Work out the finished part from the listing and answer in its coordinate system (mm). Coordinates: 2 decimals unless noted, no trailing zeros. Order: outer loops, then holes, each group sorted by start corner. A loop starts at its lowest first (then second) coordinate and runs counter-clockwise, first axis right, second up. Notation, with made-up numbers: M 50.5,-8.5 L 94.5,-8.5 A21 ccw 94.5,5.5 Z; hole C 38.5,87 d6. An arc over 180 degrees is marked long. Use a Markdown table: item, result.
from build123d import *

# Parameters (mm, degrees)
SKETCH1_W                = 110
SKETCH1_H                = 190
BOSS_EXTRUDE1_DEPTH      = 6
CUT_EXTRUDE1_REACH       = 111.936
SKETCH2_R                = 13
CUT_EXTRUDE2_REACH       = 111.936
SKETCH3_R                = 4.1
FILLET1_R                = 3
M4_CLEARANCE_HOLE1_D     = 4.2
M4_CLEARANCE_HOLE1_DEPTH = 19.75
M4_CLEARANCE_HOLE1_TIP   = 1.2618073


with BuildPart() as part:
    # Sketch1 → Boss-Extrude1 (new body)
    with BuildSketch(Plane.XY):
        Rectangle(SKETCH1_W, SKETCH1_H)
    extrude(amount=BOSS_EXTRUDE1_DEPTH)

    # Sketch2 → Cut-Extrude1 (cut, up to next)
    with BuildSketch(Plane.XY.offset(6), mode=Mode.PRIVATE) as cut_extrude1_sk1:
        Circle(SKETCH2_R)
    cut_extrude1_tool1 = extrude(cut_extrude1_sk1.sketch, amount=-CUT_EXTRUDE1_REACH, mode=Mode.PRIVATE) & part.part
    add(cut_extrude1_tool1.solids().sort_by_distance((0, 0, 6))[0], mode=Mode.SUBTRACT)

    # Sketch3 → Cut-Extrude2 (cut, up to next)
    with BuildSketch(Plane.XY.offset(6), mode=Mode.PRIVATE) as cut_extrude2_sk1:
        with Locations((-35, 75)):
            Circle(SKETCH3_R)
    cut_extrude2_tool1 = extrude(cut_extrude2_sk1.sketch, amount=-CUT_EXTRUDE2_REACH, mode=Mode.PRIVATE) & part.part
    # Sketch3 → Cut-Extrude2 (cut, up to next)
    with BuildSketch(Plane.XY.offset(6), mode=Mode.PRIVATE) as cut_extrude2_sk2:
        with Locations((35, 75)):
            Circle(SKETCH3_R)
    cut_extrude2_tool2 = extrude(cut_extrude2_sk2.sketch, amount=-CUT_EXTRUDE2_REACH, mode=Mode.PRIVATE) & part.part
    # Sketch3 → Cut-Extrude2 (cut, up to next)
    with BuildSketch(Plane.XY.offset(6), mode=Mode.PRIVATE) as cut_extrude2_sk3:
        with Locations((35, -75)):
            Circle(SKETCH3_R)
    cut_extrude2_tool3 = extrude(cut_extrude2_sk3.sketch, amount=-CUT_EXTRUDE2_REACH, mode=Mode.PRIVATE) & part.part
    # Sketch3 → Cut-Extrude2 (cut, up to next)
    with BuildSketch(Plane.XY.offset(6), mode=Mode.PRIVATE) as cut_extrude2_sk4:
        with Locations((-35, -75)):
            Circle(SKETCH3_R)
    cut_extrude2_tool4 = extrude(cut_extrude2_sk4.sketch, amount=-CUT_EXTRUDE2_REACH, mode=Mode.PRIVATE) & part.part
    add(cut_extrude2_tool1.solids().sort_by_distance((-35, 75, 6))[0], mode=Mode.SUBTRACT)
    add(cut_extrude2_tool2.solids().sort_by_distance((35, 75, 6))[0], mode=Mode.SUBTRACT)
    add(cut_extrude2_tool3.solids().sort_by_distance((35, -75, 6))[0], mode=Mode.SUBTRACT)
    add(cut_extrude2_tool4.solids().sort_by_distance((-35, -75, 6))[0], mode=Mode.SUBTRACT)

    # Fillet1
    fillet1_edges = [part.edges().sort_by_distance(p)[0] for p in [
        (55, -95, 3),
        (-55, -95, 3),
        (-55, 95, 3),
        (55, 95, 3),
    ]]
    fillet(fillet1_edges, radius=FILLET1_R)

    # M4 Clearance Hole1
    with Locations(Plane(origin=(-12, 12, 6), x_dir=(1, 0, 0), z_dir=(0, 0, 1))):
        with Locations((0, 0), (24, 0), (24, -24), (0, -24)):
            Hole(M4_CLEARANCE_HOLE1_D / 2, depth=M4_CLEARANCE_HOLE1_DEPTH)
            with Locations((0, 0, -(M4_CLEARANCE_HOLE1_DEPTH + M4_CLEARANCE_HOLE1_TIP / 2))):  # 118° drill point
                Cone(0, M4_CLEARANCE_HOLE1_D / 2, M4_CLEARANCE_HOLE1_TIP, mode=Mode.SUBTRACT)


solid = part.part
1. For a pull along X with two mould halves and no side action, classify faces 1 (the face through (-1, 22, 0)), 2 (the face through (-55, -1, 3)), 3 (the face through (-10.316, -7.91, 3.042)) as +X half, -X half, draft (parallel to the pull), parting line (faces both ways), or undercut.
Answers below:
| item | result |
|---|---|
| face 1 | draft |
| face 2 | -X half |
| face 3 | undercut |
2. Section A-A on x = 0 is taken. Determine the outline of the cut face in (y, z).
Answers below:
| item | result |
|---|---|
| outline | M -95,0 L -13,0 L -13,6 L -95,6 Z; M 13,0 L 95,0 L 95,6 L 13,6 Z |
3. Section B-B on y = 75 is taken. Determine the outline of the cut face in (x, z), then the cut area to 3 significant figures.
Answers below:
| item | result |
|---|---|
| outline | M -55,0 L -39.1,0 L -39.1,6 L -55,6 Z; M -30.9,0 L 30.9,0 L 30.9,6 L -30.9,6 Z; M 39.1,0 L 55,0 L 55,6 L 39.1,6 Z |
| area | 562 mm² |
4. Section D-D on y = 0 is taken. Determine the outline of the cut face in (x, z).
Answers below:
| item | result |
|---|---|
| outline | M -55,0 L -13,0 L -13,6 L -55,6 Z; M 13,0 L 55,0 L 55,6 L 13,6 Z |
5. Section C-C on z = 2.45 is taken. Give the number of separate pieces and of enclosed holes in the cut face, then the cut area to 3 significant figures.
Answers below:
| item | result |
|---|---|
| separate pieces | 1 |
| enclosed holes | 9 |
| area | 20,100 mm² |
6. Flat-ended cylindrical pins translate along their axes: P1, Ø7.5, axis at x = 35, y = 75, coming from the -Z side; P2, Ø8, axis at x = -40, y = -13, coming from the -Z side. Find the tip coordinate at first contact, or state that the pin passes through.
Answers below:
| item | result |
|---|---|
| P1 | through |
| P2 | z = 0 |
7. Find the intervals of material crossed by probe 1 along Y at (x, z) = (-35, 1.3); probe 2 along X at (y, z) = (-77, 4.5); probe 3 along Y at (x, z) = (4, 4.05), in increasing order.
Answers below:
| item | result |
|---|---|
| probe 1 | -95 to -79.1, -70.9 to 70.9, 79.1 to 95 |
| probe 2 | -55 to -38.58, -31.42 to 31.42, 38.58 to 55 |
| probe 3 | -95 to -12.37, 12.37 to 95 |
